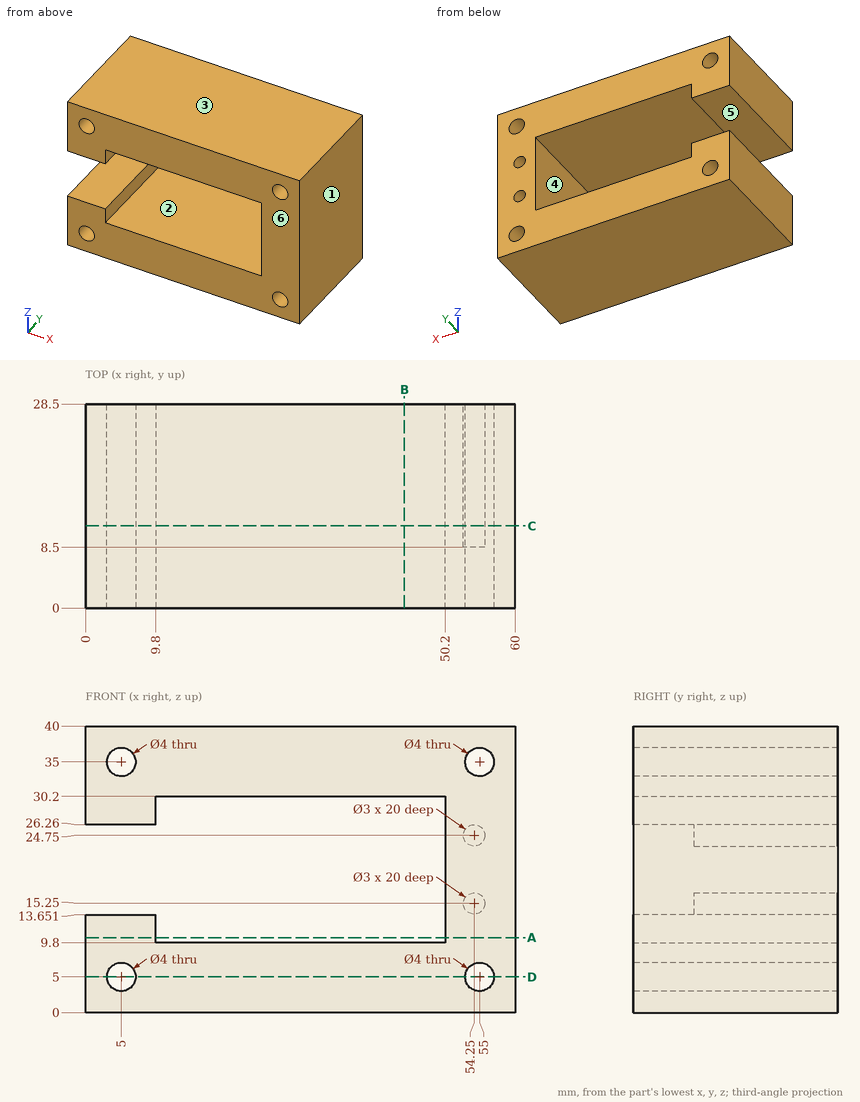
Print and shaded views of the part. All mm, measured from the part's lowest x, y and z. A direction names the side the tool comes from. Round coordinates to 2 decimals unless told otherwise and drop trailing zeros. Order: outer loops, then holes, each group sorted by start corner. A loop starts at its lowest first (then second) coordinate and runs counter-clockwise, first axis right, second up.
Q1. Two-plate mould, pull along Z, no slides. Class the marked faces 1, 2 and 3: pulls with the +Z half, pulls with the -Z half, needs draft (parallel to the pull), parting line crosses it, or undercut.
Q2. Drop flat-ended pins along their axis: pin 1 (2.5 mm diameter, centred on x = 54.25, z = 15.25, fed in from +Y); pin 2 (2.5 mm diameter, centred on x = 5, z = 5, fed in from -Y); pin 3 (10 mm diameter, centred on y = 16, z = 20, fed in from -X). Give the stop position or say it passes through.
Q3. Slice it at A-A (z = 10.5). Write the cut outline in (x, y).
Q4. Slice it at C-C (y = 11.5). Write the cut outline in (x, z).
Q5. Slice it at B-B (x = 44.5). Write the cut outline in (y, z).
Q6. Which spindle directions (+Z, -Z, +X, -X, +Y, -Y) get a long thin tool onto all of the face, cutting with end or side? Do the marked faces 4, 5 and 6. Say none if no direction does.
Q7. Slice it at D-D (z = 5). Write the cut outline in (x, y).
Q8. Wall check: L1, parallel to Z at x = 55, y = 8; L2, parallel to Z at x = 5, y = 18; L3, parallel to Z at x = 18.5, y = 21. Give the ranges that are in metal, low to high.
Results below:
1. face 1: needs draft
1. face 2: undercut
1. face 3: pulls with the +Z half
2. pin 1: stops at y = 8.5
2. pin 2: passes through
2. pin 3: stops at x = 50.2
3. outline: (0, 0) - (9.8, 0) - (9.8, 28.5) - (0, 28.5) - close; (50.2, 0) - (60, 0) - (60, 28.5) - (50.2, 28.5) - close
4. outline: (0, 0) - (60, 0) - (60, 40) - (0, 40) - (0, 26.26) - (9.8, 26.26) - (9.8, 30.2) - (50.2, 30.2) - (50.2, 9.8) - (9.8, 9.8) - (9.8, 13.65) - (0, 13.65) - close; hole circle Ø4 at (5, 5); hole circle Ø4 at (5, 35); hole circle Ø3 at (54.25, 15.25); hole circle Ø3 at (54.25, 24.75); hole circle Ø4 at (55, 5); hole circle Ø4 at (55, 35)
5. outline: (0, 0) - (28.5, 0) - (28.5, 9.8) - (0, 9.8) - close; (0, 30.2) - (28.5, 30.2) - (28.5, 40) - (0, 40) - close
6. face 4: +Y, -Y
6. face 5: -X, +Y, -Y
6. face 6: +Z, -Z, +X, -X, -Y
7. outline: (0, 0) - (3, 0) - (3, 28.5) - (0, 28.5) - close; (7, 0) - (53, 0) - (53, 28.5) - (7, 28.5) - close; (57, 0) - (60, 0) - (60, 28.5) - (57, 28.5) - close
8. L1: z = 0 to 3, 7 to 33, 37 to 40
8. L2: z = 0 to 3, 7 to 13.65, 26.26 to 33, 37 to 40
8. L3: z = 0 to 9.8, 30.2 to 40
